Check sheet for the drawn part. Datum: minimum x, y, z corner. Units: mm. Give positions to 0.01 mm unless a question says otherwise; leave off trailing zeros. Loops run counter-clockwise (first coordinate to the right, second up) from the corner with the lowest first, then second, coordinate; pieces in that order, holes last. Notation, with made-up numbers: (-26, 39.25) - (3, 39.25) arc R23 cw to (3, 69.25) - close; hole circle Ø10 at (62, -10.75). An arc over 180 degrees is marked (long way). Use a Markdown table: item, result. Add a question column.
1. Material ranges on L1, parallel to Z at x = 25.4, y = 7 (3 decimals); L2, parallel to Z at x = 330.2, y = 15.75 (3 decimals); L3, parallel to X at y = 15, z = 20.5, recorded low to high.
2. Cross-section at A-A on x = 210.5. Enter the section's corners in (y, z).
3. Depth check by flat-ended pin: P1, Ø4.5, axis at x = 25.4, z = 22.225, coming from the +Y side; P2, Ø2.5, axis at x = 147, y = 16, coming from the +Z side. Enter the tip coordinate at first touch or a pass-through.
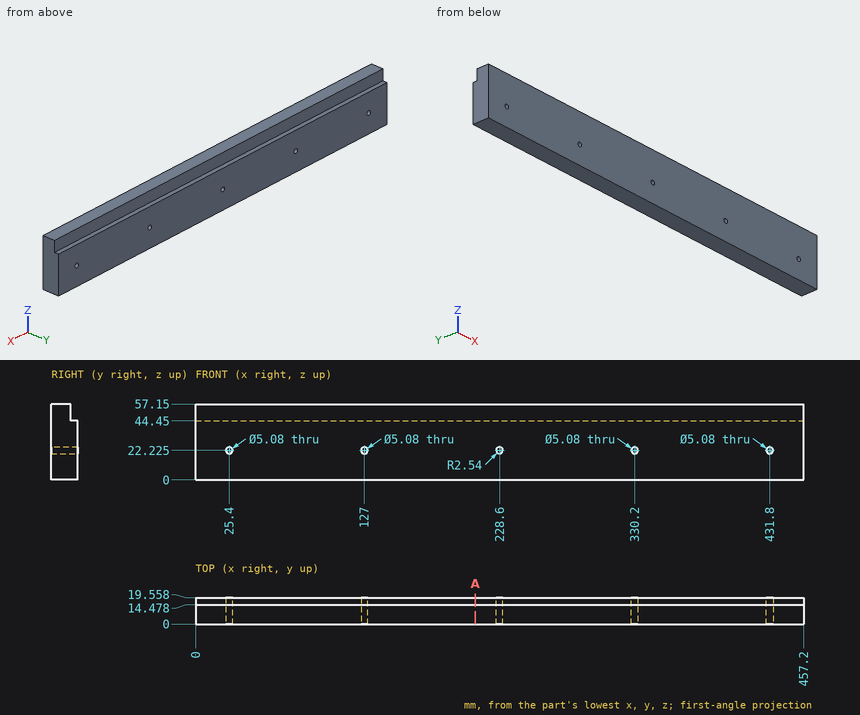
Values found:
| question | item | result |
|---|---|---|
| 1 | L1 | z = 0 to 19.685, 24.765 to 57.15 |
| 1 | L2 | z = 0 to 19.685, 24.765 to 44.45 |
| 1 | L3 | x = 0 to 23.54, 27.26 to 125.14, 128.86 to 226.74, 230.46 to 328.34, 332.06 to 429.94, 433.66 to 457.2 |
| 2 | outline | (0, 0) - (19.56, 0) - (19.56, 44.45) - (14.48, 44.45) - (14.48, 57.15) - (0, 57.15) - close |
| 3 | P1 | passes through |
| 3 | P2 | stops at z = 44.45 |
